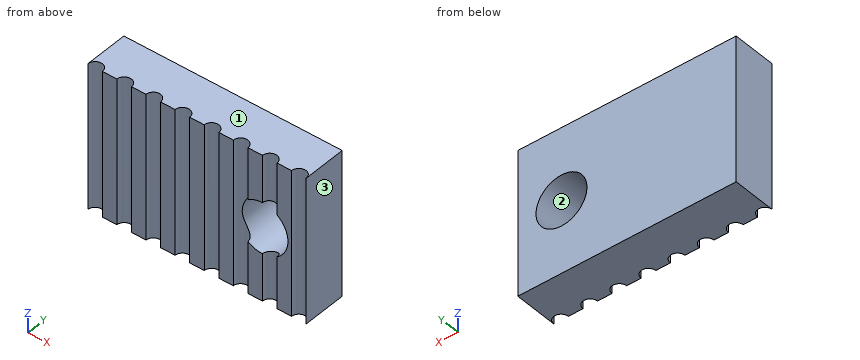
from build123d import *

# Parameters (mm, degrees)
SKETCH1_W           = 15
SKETCH1_H           = 10
BOSS_EXTRUDE1_DEPTH = 3
SKETCH2_R           = 1.75
CUT_EXTRUDE1_DEPTH  = 10.5
CUT_EXTRUDE2_DEPTH  = 13.854960132
LPATTERN1_COUNT     = 7
LPATTERN1_PITCH     = 2


with BuildPart() as part:
    # Sketch1 → Boss-Extrude1 (new body)
    with BuildSketch(Plane(origin=(0, 0, 0), x_dir=(1, 0, 0), z_dir=(0, 1, 0))):
        Rectangle(SKETCH1_W, SKETCH1_H)
    extrude(amount=BOSS_EXTRUDE1_DEPTH)

    # Sketch2 → Cut-Extrude1 (cut, through all)
    with BuildSketch(Plane(origin=(0, 3, 0), x_dir=(1, 0, 0), z_dir=(0, 1, 0))):
        with Locations(Location((4.5, 0, 0), (0, 0, 270))):
            Circle(SKETCH2_R)
    extrude(amount=-CUT_EXTRUDE1_DEPTH, mode=Mode.SUBTRACT)

    # Sketch3 → Cut-Extrude2 (cut, through all)
    with BuildSketch(Plane.XY.offset(5)):
        with BuildLine():
            Line((-7.5, 0), (-6.5, 0))
            ThreePointArc((-6.5, 0), (-7, 0.5), (-7.5, 0))
        make_face()
        with BuildLine():
            Line((-5.5, 0), (-4.5, 0))
            ThreePointArc((-4.5, 0), (-5, 0.5), (-5.5, 0))
        make_face()
    cut_extrude2 = extrude(amount=-CUT_EXTRUDE2_DEPTH, mode=Mode.SUBTRACT)

    # LPattern1: Cut-Extrude2 ×7
    with Locations(*[(i * LPATTERN1_PITCH, 0, 0) for i in range(1, LPATTERN1_COUNT)]):
        add(cut_extrude2, mode=Mode.SUBTRACT)


solid = part.part
Can you work these out from the model? Positions are in its coordinate system, mm. Face numbers are marked on the shaded views. Give positions to 0.01 mm unless a question says otherwise; leave off trailing zeros. Loops run counter-clockwise (first coordinate to the right, second up) from the corner with the lowest first, then second, coordinate; pieces in that order, holes last. Notation, with made-up numbers: (-0.5, 41) - (4.5, 41) arc R19 cw to (4.5, 76) - close; hole circle Ø10 at (67.25, 51.5). An arc over 180 degrees is marked (long way). Answer as a JSON object with one key per item and string values.
Q1. Will this pin go through, and if not, where does the flat tip stop? P1, Ø5, axis at x = -2.5, z = -1, coming from the -Y side.
Geometry says:
{"P1": "y = 0"}
Q2. Imagine slicing it at C-C on z = 0.75. Write out the boundary of the cut face in (x, y).
Geometry says:
{"outline": "(-7.5, 0) arc R0.5 cw to (-6.5, 0) - (-5.5, 0) arc R0.5 cw to (-4.5, 0) - (-3.5, 0) arc R0.5 cw to (-2.5, 0) - (-1.5, 0) arc R0.5 cw to (-0.5, 0) - (0.5, 0) arc R0.5 cw to (1.5, 0) - (2.5, 0) arc R0.5 cw to (2.92, 0.49) - (2.92, 3) - (-7.5, 3) - close; (6.08, 0) - (6.5, 0) arc R0.5 cw to (7.5, 0) - (7.5, 3) - (6.08, 3) - close"}
Q3. Imagine slicing it at D-D on z = 4.25. Write out the boundary of the cut face in (x, y).
Geometry says:
{"outline": "(-7.5, 0) arc R0.5 cw to (-6.5, 0) - (-5.5, 0) arc R0.5 cw to (-4.5, 0) - (-3.5, 0) arc R0.5 cw to (-2.5, 0) - (-1.5, 0) arc R0.5 cw to (-0.5, 0) - (0.5, 0) arc R0.5 cw to (1.5, 0) - (2.5, 0) arc R0.5 cw to (3.5, 0) - (4.5, 0) arc R0.5 cw to (5.5, 0) - (6.5, 0) arc R0.5 cw to (7.5, 0) - (7.5, 3) - (-7.5, 3) - close"}
Q4. If I drill on L1, parallel to X at y = 2.25, z = 0; L2, parallel to Z at x = 4.5, y = 2.2; L3, parallel to Y at x = 5, z = -3.5, over which ranges is the centre line in solid material (lowest first)?
Geometry says:
{"L1": "-7.5 to 2.75, 6.25 to 7.5", "L2": "-5 to -1.75, 1.75 to 5", "L3": "0.5 to 3"}
Q5. Imagine slicing it at B-B on y = 2.5. Write out the boundary of the cut face in (x, z).
Geometry says:
{"outline": "(-7.5, -5) - (7.5, -5) - (7.5, 5) - (-7.5, 5) - close; hole circle Ø3.5 at (4.5, 0)"}
Q6. Imagine slicing it at A-A on x = 3. Write out the boundary of the cut face in (y, z).
Geometry says:
{"outline": "(0.5, -5) - (3, -5) - (3, -0.9) - (0.5, -0.9) - close; (0.5, 0.9) - (3, 0.9) - (3, 5) - (0.5, 5) - close"}
Q7. If we mould it in two halves opening along Z, with no side actions, what happens to the marked faces 1, 2 and 3? For each: pulls with the +Z half, pulls with the -Z half, needs draft (parallel to the pull), parting line crosses it, or undercut.
Geometry says:
{"face 1": "pulls with the +Z half", "face 2": "undercut", "face 3": "needs draft"}
